Design review of the part built by this model. Coordinates are the model's own, in mm. A direction names the side the tool comes from. Give positions to 0.01 mm unless a question says otherwise; leave off trailing zeros. Loops run counter-clockwise (first coordinate to the right, second up) from the corner with the lowest first, then second, coordinate; pieces in that order, holes last. Notation, with made-up numbers: (61, 11) -> (103, 11) arc R35 cw to (103, 49) -> close; hole circle Ø4 at (31.5, -4.75). An arc over 180 degrees is marked (long way). Use CSV: the item, a comma, the result in double quotes. Start each with the question number.
Item 1: We need section B-B (z = -64). State the section outline as (x, y) points.
Item 2: We need section C-C (x = -11). State the section outline as (y, z) points, plus the area to 3 significant figures.
Item 3: The part is to be moulded in two halves that separate along Z. For faces 1 (the face through (-12.5, 12, -35)), 2 (the face through (-39.274, 4.174, -12.215)), say which applies: +Z half, -Z half, draft (parallel to the pull), parting line (faces both ways), or undercut.
Item 4: For faces 3 (the face through (-42, 5, -23)), 4 (the face through (-8, 5, -27)), 5 (the face through (-39.72, 5.06, -43.65)), list the 3-axis set-ups (+Z, -Z, +X, -X, +Y, -Y) from which the entire face can be reached by the end or side of a thin tool; tool diameter is ignored.
Item 5: We need section A-A (y = 12.75). State the section outline as (x, z) points.
Item 6: We need section D-D (z = -31.5). State the section outline as (x, y) points, plus the area to 3 significant figures.
Item 7: Wall thickness on line 1 along Y through (x, z) = (-10, -25); line 2 along Y through (x, z) = (-47.5, -45); line 3 along X through (y, z) = (22.25, -36): over which ranges is each line inside the solid? List them lowest first. Write a range as from..to.
Item 8: Clearance check with flat-ended pins moving along their axes: pin 1 (1.5 mm diameter, centred on y = 19, z = -17.5, fed in from +X); pin 2 (6 mm diameter, centred on x = -44.5, y = 11, fed in from +Z); pin 3 (2.5 mm diameter, centred on y = 18, z = -44.5, fed in from -X); pin 4 (7 mm diameter, centred on y = 5, z = -25, fed in from +X). State where each tip first meets the part, or that it passes through.
Autodesk Inventor part; units mm, degrees
ref_plane "YZ Plane" through (0, 0, 0) normal (1, 0, 0) x (0, 1, 0)
ref_plane "XZ Plane" through (0, 0, 0) normal (0, 1, 0) x (-1, 0, 0)
ref_plane "XY Plane" through (0, 0, 0) normal (0, 0, 1) x (1, 0, 0)
sketch "スケッチ1" plane through (0, 0, 0) normal (0, 1, 0) x (-1, 0, 0)
  line L0 (0, 0) -> (50, 0)
  line L1 (50, 0) -> (50, -75)
  line L2 (50, -75) -> (0, -75)
  line L3 (0, -75) -> (0, 0)
  dimension "d0" = 50
  dimension "d1" = 75
extrude "押し出し1" add sketch "スケッチ1" along normal blind 29
sketch "スケッチ2" plane through (0, 0, 0) normal (0, -1, 0) x (1, 0, 0)
  line L0 (-50, 0) -> (0, 0)
  line L1 (0, -75) -> (-50, -75)
  line L2 (-37.5, 0) -> (-12.5, 0)
  line L3 (-12.5, 0) -> (-12.5, -75)
  line L4 (-12.5, -75) -> (-37.5, -75)
  line L5 (-37.5, -75) -> (-37.5, 0)
  line L6 (-50, 0) -> (0, 0)
  point P0 (-12.5, -37.5)
  point P1 (-25, 0)
  point P2 (-25, 0)
  dimension "d4" = 25
extrude "押し出し2" cut sketch "スケッチ2" against normal blind 25
sketch "スケッチ3" plane through (0, 0, 0) normal (1, 0, 0) x (0, 0, -1)
  line L0 (0, 0) -> (20, 0)
  line L1 (20, 0) -> (20, 25)
  line L2 (20, 25) -> (0, 25)
  line L3 (0, 25) -> (0, 0)
  line L4 (50, 0) -> (70, 0)
  line L5 (70, 0) -> (70, 25)
  line L6 (70, 25) -> (50, 25)
  line L7 (50, 25) -> (50, 0)
  line L8 (0, 25) -> (75, 25)
  point P0 (60, 25)
  point P1 (10, 25)
  dimension "d7" = 20
  dimension "d8" = 20
  dimension "d9" = 50
extrude "押し出し3" cut sketch "スケッチ3" against normal up to surface (12.5 mm away)
sketch "スケッチ4" plane through (-50, 0, -75) normal (-1, 0, 0) x (0, 0, 1)
  circle A0 centre (62, 20.5) radius 0.85
  circle A1 centre (62, 4.5) radius 0.85
  circle A2 centre (11, 4.5) radius 0.85
  line L0 (62, 20.5) -> (62, 4.5) construction
  line L1 (62, 4.5) -> (11, 4.5) construction
  line L2 (75, 0) -> (75, 25)
  point P0 (75, 12.5)
  point P1 (62, 12.5)
  dimension "d12" = 1.7
  dimension "d13" = 1.7
  dimension "d14" = 1.7
  dimension "d15" = 16
  dimension "d16" = 51
  dimension "d17" = 13
extrude "押し出し4" cut sketch "スケッチ4" against normal up to surface (12.5 mm away)
sketch "スケッチ5" plane through (-50, 0, -75) normal (-1, 0, 0) x (0, 0, 1)
  circle A0 centre (11, 4.5) radius 0.85
  circle A1 centre (11, 4.5) radius 4
  circle A2 centre (62, 20.5) radius 0.85
  circle A3 centre (62, 20.5) radius 4
  circle A4 centre (62, 4.5) radius 0.85
  circle A5 centre (62, 4.5) radius 4
  point P0 (75, 0)
  dimension "d20" = 8
  dimension "d21" = 8
  dimension "d22" = 8
extrude "押し出し5" cut sketch "スケッチ5" against normal blind 9
fillet "フィレット1" radius 10 2 edges at (-43.75, 0, 0) (-43.75, 0, -75)
sketch "スケッチ7" plane through (0, 0, -75) normal (1, 0, 0) x (0, 0, -1)
  line L0 (-30, 5) -> (-50, 5) construction
  line L1 (-50, 5) -> (-50, 19) construction
  line L2 (-50, 19) -> (-30, 19) construction
  line L3 (-30, 19) -> (-30, 5) construction
  line L4 (-55, 0) -> (-25, 0)
  line L5 (-25, 0) -> (-25, 25)
  line L6 (-55, 25) -> (-55, 0)
  line L7 (-75, 29) -> (0, 29)
  circle A0 centre (-50, 5) radius 1.35
  circle A1 centre (-30, 5) radius 1.35
  circle A2 centre (-30, 19) radius 1.35
  circle A3 centre (-50, 19) radius 1.35
  point P0 (-75, 0)
  dimension "d26" = 5
  dimension "d27" = 5
  dimension "d28" = 5
  dimension "d29" = 10
  dimension "d30" = 2.7
  dimension "d31" = 2.7
  dimension "d32" = 2.7
  dimension "d33" = 2.7
extrude "押し出し6" cut sketch "スケッチ7" against normal through all
fillet "フィレット2" radius 20 1 edges at (0, 27, 0)
sketch "スケッチ8" plane through (0, 0, -75) normal (1, 0, 0) x (0, 0, -1)
  circle A0 centre (-30, 19) radius 4
  circle A1 centre (-30, 5) radius 4
  circle A2 centre (-50, 5) radius 4
  circle A3 centre (-50, 19) radius 4
  circle A4 centre (-30, 5) radius 1.35
  circle A5 centre (-30, 19) radius 1.35
  circle A6 centre (-50, 19) radius 1.35
  circle A7 centre (-50, 5) radius 1.35
  point P0 (-75, 0)
  dimension "d37" = 8
  dimension "d38" = 8
  dimension "d39" = 8
  dimension "d40" = 8
extrude "押し出し7" cut sketch "スケッチ8" against normal blind 8 contours A0 | A1 | A2 | A3 | A4 | A5 | A6 | A7
sketch "スケッチ9" plane through (-50, 29, -75) normal (-1, 0, 0) x (0, 0, 1)
  circle A0 centre (30, -24) radius 4
  circle A1 centre (30, -10) radius 4
  circle A2 centre (50, -24) radius 4
  circle A3 centre (50, -10) radius 4
  circle A4 centre (30, -10) radius 1.35
  circle A5 centre (30, -24) radius 1.35
  circle A6 centre (50, -10) radius 1.35
  circle A7 centre (50, -24) radius 1.35
  point P0 (75, -29)
  dimension "d43" = 8
  dimension "d44" = 8
  dimension "d45" = 8
  dimension "d46" = 8
extrude "押し出し8" cut sketch "スケッチ9" against normal blind 8 contours A0 | A1 | A2 | A3 | A4 | A5 | A6 | A7
sketch "スケッチ11" plane through (0, 29, 0) normal (0, 1, 0) x (1, 0, 0)
  line L0 (-49.5, 90) -> (-0.5, 90)
  line L1 (-0.5, 90) -> (-0.5, -10)
  line L2 (-0.5, -10) -> (-49.5, -10)
  line L3 (-49.5, -10) -> (-49.5, 90)
  line L4 (-50, 75) -> (-50, 0)
  line L5 (0, 20) -> (0, 75)
  line L6 (-80, 110) -> (50, 110)
  line L7 (50, 110) -> (50, -10)
  line L8 (50, -10) -> (-80, -10)
  line L9 (-80, -10) -> (-80, 110)
  point P0 (0, 0)
  point P1 (-0.5, -10)
  dimension "d49" = 0.5
  dimension "d50" = 0.5
extrude "押し出し9" cut sketch "スケッチ11" against normal through all contours L3 L8 L9 L6 L7 L1 L0
equation "\"d8\" = d7"
properties part number "モーター接続"
Results found:
1,outline,"(-49.5, 0) -> (-37.5, 0) -> (-37.5, 3.65) -> (-41, 3.65) -> (-41, 0.5) -> (-49.5, 0.5) -> close; (-49.5, 8.5) -> (-41, 8.5) -> (-41, 5.35) -> (-37.5, 5.35) -> (-37.5, 25) -> (-0.5, 25) -> (-0.5, 29) -> (-49.5, 29) -> close"
2,outline,"(0, -75) -> (29, -75) -> (29, -2.14) -> (25, -2.14) -> (25, -20) -> (0, -20) -> (0, -50) -> (25, -50) -> (25, -70) -> (0, -70) -> close; hole circle Ø2.7 at (5, -45); hole circle Ø2.7 at (5, -25); hole circle Ø2.7 at (19, -45); hole circle Ø2.7 at (19, -25)"
2,area,"1,140 mm²"
3,face 1,"draft"
3,face 2,"undercut"
4,face 3,"-X"
4,face 4,"+X"
4,face 5,"+X, -X"
5,outline,"(-49.5, -75) -> (-37.5, -75) -> (-37.5, 0) -> (-49.5, 0) -> close; (-12.5, -75) -> (-0.5, -75) -> (-0.5, -70) -> (-12.5, -70) -> close; (-12.5, -50) -> (-0.5, -50) -> (-0.5, -20) -> (-12.5, -20) -> close"
6,outline,"(-49.5, 0) -> (-37.5, 0) -> (-37.5, 25) -> (-12.5, 25) -> (-12.5, 0) -> (-0.5, 0) -> (-0.5, 29) -> (-49.5, 29) -> close"
6,area,"796 mm²"
7,line 1,"0..3.65, 6.35..17.65, 20.35..29"
7,line 2,"0..1, 9..15, 23..29"
7,line 3,"-49.5..-37.5, -12.5..-0.5"
8,pin 1,"x = -37.5"
8,pin 2,"z = 0"
8,pin 3,"x = -42"
8,pin 4,"x = -8"
